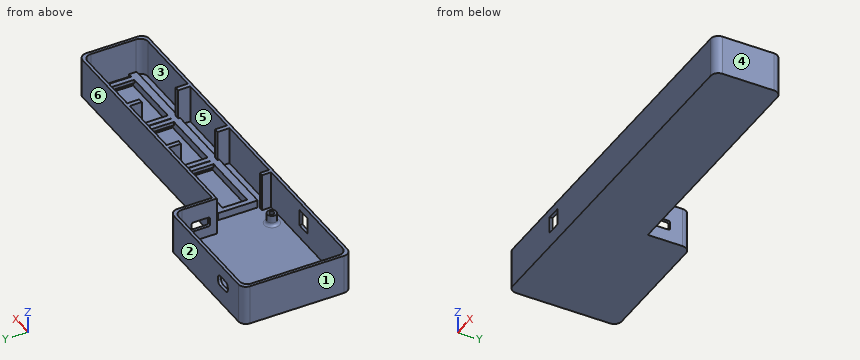
```python
from build123d import *

# Parameters (mm, degrees)
EXTRUDE_1_DEPTH     = 1.5
EXTRUDE_2_DEPTH     = 25
FILLET_1_R          = 5
SKETCH_3_R          = 3
SKETCH_3_R_2        = 1.5
EXTRUDE_3_DEPTH     = 7
FILLET_2_R          = 2
CUT_EXTRUDE_1_REACH = 182.017
SKETCH_4_W          = 6.382937609
SKETCH_4_H          = 12
FILLET_3_R          = 1
CUT_EXTRUDE_2_REACH = 256.311
SKETCH_5_W          = 11.6
SKETCH_5_H          = 7
FILLET_4_R          = 2.5
SKETCH_6_W          = 145
SKETCH_6_H          = 5
EXTRUDE_4_DEPTH     = 5
EXTRUDE_5_REACH     = 249.47
CUT_EXTRUDE_3_REACH = 256.311
SKETCH_8_W          = 9.5
SKETCH_8_H          = 11
SKETCH_9_W          = 3
SKETCH_9_H          = 8
SKETCH_9_W_2        = 2.5
SKETCH_9_H_2        = 6
EXTRUDE_6_DEPTH     = 25


with BuildPart() as part:
    # 草图1 → 凸台-拉伸1 (new body)
    with BuildSketch(Plane.XY):
        Polygon((104.053507175, -78.126332489), (-4.538088534, -78.126332489), (-4.538088534, -6.126332489), (82.461911466, -6.126332489), (82.461911466, -34.126332489), (242.461911466, -34.126332489), (242.461911466, -78.126332489), align=None)
    extrude(amount=EXTRUDE_1_DEPTH)

    # 草图2 → 凸台-拉伸2 (add)
    with BuildSketch(Plane.XY.offset(1.5)):
        Polygon((-4.538088534, -6.126332489), (-4.538088534, -78.126332489), (242.461911466, -78.126332489), (242.461911466, -34.126332489), (82.461911466, -34.126332489), (82.461911466, -6.126332489), align=None)
        Polygon((80.461911466, -8.126332489), (-2.538088534, -8.126332489), (-2.538088534, -76.126332489), (240.461911466, -76.126332489), (240.461911466, -36.126332489), (80.461911466, -36.126332489), align=None, mode=Mode.SUBTRACT)
    extrude(amount=EXTRUDE_2_DEPTH)

    # 圆角1
    fillet_1_edges = [part.edges().sort_by_distance(p)[0] for p in [
        (-4.538088534, -6.126332489, 13.25),
        (82.461911466, -6.126332489, 13.25),
        (242.461911466, -34.126332489, 13.25),
        (242.461911466, -78.126332489, 13.25),
        (-4.538088534, -78.126332489, 13.25),
        (80.461911466, -8.126332489, 14),
        (-2.538088534, -8.126332489, 14),
        (-2.538088534, -76.126332489, 14),
        (240.461911466, -76.126332489, 14),
        (240.461911466, -36.126332489, 14),
    ]]
    fillet(fillet_1_edges, radius=FILLET_1_R)

    # 草图3 → 凸台-拉伸3 (add)
    # profile 1 of 4: a face of its own
    with BuildSketch(Plane.XY.offset(1.5)):
        with Locations((74.461811484, -14.126255575)):
            Circle(SKETCH_3_R)
        with Locations((74.461811484, -14.126255575)):
            Circle(SKETCH_3_R_2, mode=Mode.SUBTRACT)
    # profile 2 of 4: a face of its own
    with BuildSketch(Plane.XY.offset(1.5)):
        with Locations((4.461811484, -14.126255575)):
            Circle(SKETCH_3_R)
        with Locations((4.461811484, -14.126255575)):
            Circle(SKETCH_3_R_2, mode=Mode.SUBTRACT)
    # profile 3 of 4: a face of its own
    with BuildSketch(Plane.XY.offset(1.5)):
        with Locations((4.461811484, -69.126255575)):
            Circle(SKETCH_3_R)
        with Locations((4.461811484, -69.126255575)):
            Circle(SKETCH_3_R_2, mode=Mode.SUBTRACT)
    # profile 4 of 4: a face of its own
    with BuildSketch(Plane.XY.offset(1.5)):
        with Locations((74.461811484, -69.126255575)):
            Circle(SKETCH_3_R)
        with Locations((74.461811484, -69.126255575)):
            Circle(SKETCH_3_R_2, mode=Mode.SUBTRACT)
    extrude(amount=EXTRUDE_3_DEPTH)

    # 圆角2
    fillet_2_edges = [part.edges().sort_by_distance(p)[0] for p in [
        (71.461811484, -69.126255575, 1.5),
        (1.461811484, -69.126255575, 1.5),
        (1.461811484, -14.126255575, 1.5),
        (71.461811484, -14.126255575, 1.5),
    ]]
    fillet(fillet_2_edges, radius=FILLET_2_R)

    # 草图4 → 切除-拉伸1 (cut, up to next)
    with BuildSketch(Plane(origin=(82.461911466, 0, 0), x_dir=(0, 0, -1), z_dir=(1, 0, 0)), mode=Mode.PRIVATE) as cut_extrude_1_sk1:
        with Locations((-11.691468805, -25.526333622)):
            Rectangle(SKETCH_4_W, SKETCH_4_H)
    cut_extrude_1_tool1 = extrude(cut_extrude_1_sk1.sketch, amount=-CUT_EXTRUDE_1_REACH, mode=Mode.PRIVATE) & part.part
    add(cut_extrude_1_tool1.solids().sort_by_distance((82.461911, -25.526334, 11.691469))[0], mode=Mode.SUBTRACT)

    # 圆角3
    fillet_3_edges = [part.edges().sort_by_distance(p)[0] for p in [
        (81.461911466, -19.526333622, 8.5),
        (81.461911466, -31.526333622, 8.5),
        (81.461911466, -31.526333622, 14.882937609),
        (81.461911466, -19.526333622, 14.882937609),
    ]]
    fillet(fillet_3_edges, radius=FILLET_3_R)

    # 草图5 → 切除-拉伸2 (cut, up to next)
    with BuildSketch(Plane(origin=(0, -6.126332489, 0), x_dir=(1, 0, 0), z_dir=(0, 1, 0)), mode=Mode.PRIVATE) as cut_extrude_2_sk1:
        with Locations((18.833572944, -15.2)):
            Rectangle(SKETCH_5_W, SKETCH_5_H)
    cut_extrude_2_tool1 = extrude(cut_extrude_2_sk1.sketch, amount=-CUT_EXTRUDE_2_REACH, mode=Mode.PRIVATE) & part.part
    add(cut_extrude_2_tool1.solids().sort_by_distance((18.833573, -6.126332, 15.2))[0], mode=Mode.SUBTRACT)

    # 圆角4
    fillet_4_edges = [part.edges().sort_by_distance(p)[0] for p in [
        (24.633572944, -7.126332489, 11.7),
        (24.633572944, -7.126332489, 18.7),
        (13.033572944, -7.126332489, 18.7),
        (13.033572944, -7.126332489, 11.7),
    ]]
    fillet(fillet_4_edges, radius=FILLET_4_R)

    # 草图6 → 凸台-拉伸4 (add)
    with BuildSketch(Plane.XY.offset(1.5)):
        with Locations((164.146026619, -45.476332489)):
            Rectangle(SKETCH_6_W, SKETCH_6_H)
        with Locations((164.146026619, -66.776332489)):
            Rectangle(SKETCH_6_W, SKETCH_6_H)
    extrude(amount=EXTRUDE_4_DEPTH)

    # 草图7 → 凸台-拉伸5 (add, up to next)
    with BuildSketch(Plane.XZ.offset(47.976332489), mode=Mode.PRIVATE) as extrude_5_sk1:
        Polygon((91.646026619, 6.5), (95.146026619, 6.5), (95.146026619, 4.15), (93.646026619, 4.15), (93.646026619, 1.5), (91.646026619, 1.5), align=None)
    extrude_5_tool1 = extrude(extrude_5_sk1.sketch, amount=EXTRUDE_5_REACH, mode=Mode.PRIVATE) - part.part
    # 草图7 → 凸台-拉伸5 (add, up to next)
    with BuildSketch(Plane.XZ.offset(47.976332489), mode=Mode.PRIVATE) as extrude_5_sk2:
        Polygon((138.846026619, 1.5), (138.846026619, 6.5), (135.346026619, 6.5), (135.346026619, 4.15), (136.846026619, 4.15), (136.846026619, 1.5), align=None)
    extrude_5_tool2 = extrude(extrude_5_sk2.sketch, amount=EXTRUDE_5_REACH, mode=Mode.PRIVATE) - part.part
    # 草图7 → 凸台-拉伸5 (add, up to next)
    with BuildSketch(Plane.XZ.offset(47.976332489), mode=Mode.PRIVATE) as extrude_5_sk3:
        Polygon((139.146026619, 1.5), (139.146026619, 6.5), (142.646026619, 6.5), (142.646026619, 4.15), (141.146026619, 4.15), (141.146026619, 1.5), align=None)
    extrude_5_tool3 = extrude(extrude_5_sk3.sketch, amount=EXTRUDE_5_REACH, mode=Mode.PRIVATE) - part.part
    # 草图7 → 凸台-拉伸5 (add, up to next)
    with BuildSketch(Plane.XZ.offset(47.976332489), mode=Mode.PRIVATE) as extrude_5_sk4:
        Polygon((186.346026619, 1.5), (186.346026619, 6.5), (182.846026619, 6.5), (182.846026619, 4.15), (184.346026619, 4.15), (184.346026619, 1.5), align=None)
    extrude_5_tool4 = extrude(extrude_5_sk4.sketch, amount=EXTRUDE_5_REACH, mode=Mode.PRIVATE) - part.part
    # 草图7 → 凸台-拉伸5 (add, up to next)
    with BuildSketch(Plane.XZ.offset(47.976332489), mode=Mode.PRIVATE) as extrude_5_sk5:
        Polygon((186.646026619, 1.5), (186.646026619, 6.5), (190.146026619, 6.5), (190.146026619, 4.15), (188.646026619, 4.15), (188.646026619, 1.5), align=None)
    extrude_5_tool5 = extrude(extrude_5_sk5.sketch, amount=EXTRUDE_5_REACH, mode=Mode.PRIVATE) - part.part
    # 草图7 → 凸台-拉伸5 (add, up to next)
    with BuildSketch(Plane.XZ.offset(47.976332489), mode=Mode.PRIVATE) as extrude_5_sk6:
        Polygon((233.846026619, 1.5), (233.846026619, 6.5), (230.346026619, 6.5), (230.346026619, 4.15), (231.846026619, 4.15), (231.846026619, 1.5), align=None)
    extrude_5_tool6 = extrude(extrude_5_sk6.sketch, amount=EXTRUDE_5_REACH, mode=Mode.PRIVATE) - part.part
    add(extrude_5_tool1.solids().sort_by_distance((93.102126, -47.976332, 4.345333))[0])
    add(extrude_5_tool2.solids().sort_by_distance((137.389927, -47.976332, 4.345333))[0])
    add(extrude_5_tool3.solids().sort_by_distance((140.602126, -47.976332, 4.345333))[0])
    add(extrude_5_tool4.solids().sort_by_distance((184.889927, -47.976332, 4.345333))[0])
    add(extrude_5_tool5.solids().sort_by_distance((188.102126, -47.976332, 4.345333))[0])
    add(extrude_5_tool6.solids().sort_by_distance((232.389927, -47.976332, 4.345333))[0])

    # 草图8 → 切除-拉伸3 (cut, up to next)
    with BuildSketch(Plane.XZ.offset(78.126332489), mode=Mode.PRIVATE) as cut_extrude_3_sk1:
        with Locations((49.541967888, 15.57020515)):
            Rectangle(SKETCH_8_W, SKETCH_8_H)
    cut_extrude_3_tool1 = extrude(cut_extrude_3_sk1.sketch, amount=-CUT_EXTRUDE_3_REACH, mode=Mode.PRIVATE) & part.part
    add(cut_extrude_3_tool1.solids().sort_by_distance((49.541968, -78.126332, 15.570205))[0], mode=Mode.SUBTRACT)

    # 草图9 → 凸台-拉伸6 (add)
    with BuildSketch(Plane.XY.offset(1.5)):
        with Locations((139.260338635, -40.126332489)):
            Rectangle(SKETCH_9_W, SKETCH_9_H)
        with Locations((139.260338635, -72.126332489)):
            Rectangle(SKETCH_9_W, SKETCH_9_H)
        with Locations((186.260338635, -40.126332489)):
            Rectangle(SKETCH_9_W, SKETCH_9_H)
        with Locations((186.260338635, -72.126332489)):
            Rectangle(SKETCH_9_W, SKETCH_9_H)
        with Locations((89.301714301, -73.126332489)):
            Rectangle(SKETCH_9_W_2, SKETCH_9_H_2)
    extrude(amount=EXTRUDE_6_DEPTH)


solid = part.part
```
For this review, take the finished solid that the model builds, in its own axes (mm). Face numbers are marked on the shaded views. A direction names the side the tool comes from. Coordinates: 2 decimals unless noted, no trailing zeros. Write each loop counter-clockwise with the first axis right and the second up, starting at its lowest first coordinate (ties: lowest second). Pieces come first, ordered by that corner, then holes.
(1) Add section A-A on y = -25.5. Give the boundary of the cut face in (x, z).
(2) Wall thickness on probe 1 along Y at (x, z) = (155, 3); probe 2 along Y at (x, z) = (28, 17); probe 3 along X at (y, z) = (-63, 13.25): over which ranges is each line inside the solid? List them lowest first.
(3) Add section B-B on x = 146.5. Give the boundary of the cut face in (y, z).
(4) For pin 1 Ø2 at (x, y) = (57.5, -43) entering from -Z; pin 2 Ø8 at (x, y) = (160, -55) entering from +Z; pin 3 Ø3.5 at (x, y) = (74.5, -69.5) entering from +Z; pin 4 Ø1.5 at (x, z) = (170, 3.5) entering from +Y, all flat-tipped, find the tip position at first contact; note any pin that passes through.
(5) Tool access review of the marked faces 4, 5 and 6: name each direction out of +Z, -Z, +X, -X, +Y, -Y from which nothing blocks a thin tool from reaching the whole face with its end or side.
(6) The part is to be moulded in two halves that separate along Y. For the marked faces 1, 2 and 3, say which applies: +Y half, -Y half, draft (parallel to the pull), parting line (faces both ways), or undercut.
Answer sheet:
1. outline: (-4.54, 0) - (82.46, 0) - (82.46, 8.5) - (80.46, 8.5) - (80.46, 1.5) - (-2.54, 1.5) - (-2.54, 26.5) - (-4.54, 26.5) - close; (80.46, 14.88) - (82.46, 14.88) - (82.46, 26.5) - (80.46, 26.5) - close
2. probe 1: y = -78.13 to -76.13, -69.28 to -64.28, -47.98 to -42.98, -36.13 to -34.13
2. probe 2: y = -78.13 to -76.13, -8.13 to -6.13
2. probe 3: x = -4.54 to -2.54, 240.46 to 242.46
3. outline: (-78.13, 0) - (-34.13, 0) - (-34.13, 26.5) - (-36.13, 26.5) - (-36.13, 1.5) - (-42.98, 1.5) - (-42.98, 6.5) - (-47.98, 6.5) - (-47.98, 1.5) - (-64.28, 1.5) - (-64.28, 6.5) - (-69.28, 6.5) - (-69.28, 1.5) - (-76.13, 1.5) - (-76.13, 26.5) - (-78.13, 26.5) - close
4. pin 1: stops at z = 0
4. pin 2: stops at z = 1.5
4. pin 3: stops at z = 8.5
4. pin 4: stops at y = -34.13
5. face 4: +Z, -Z, +X, +Y, -Y
5. face 5: +Z
5. face 6: +Z, -Z, +X, +Y
6. face 1: draft
6. face 2: +Y half
6. face 3: undercut
